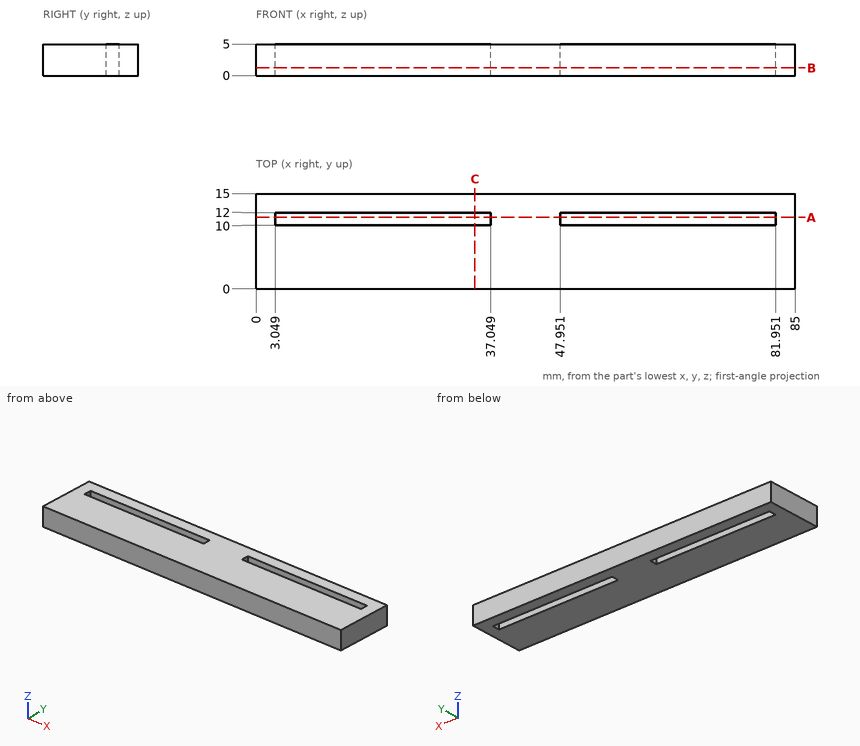
Job drawing, mm, ordinate dimensions from the low corner. One solid piece. Give positions to 0.01 mm unless a question says otherwise; leave off trailing zeros. Write each loop counter-clockwise with the first axis right and the second up, starting at its lowest first coordinate (ties: lowest second). Pieces come first, ordered by that corner, then holes. Notation, with made-up numbers: M 74.25,-35 L 90.25,-35 A22 ccw 90.25,-17 Z; hole C 22.5,65.5 d9. An arc over 180 degrees is marked long. Put each result on its own line as item: value. Start each with the question number.
(1) Band-saw the part on A-A, the plane y = 11.25. Write the cut outline in (x, z).
(2) Band-saw the part on B-B, the plane z = 1.25. Write the cut outline in (x, y).
(3) Band-saw the part on C-C, the plane x = 34.5. Write the cut outline in (y, z).
(4) Probe L1, parallel to X at y = 10.75, z = 0.7; L2, parallel to Y at x = 65, z = 1.65. List the from-to ranges inside material, lowest first.
Response values:
1. outline: M 0,0 L 3.05,0 L 3.05,5 L 0,5 Z; M 37.05,0 L 47.95,0 L 47.95,5 L 37.05,5 Z; M 81.95,0 L 85,0 L 85,5 L 81.95,5 Z
2. outline: M 0,0 L 85,0 L 85,15 L 0,15 Z; hole M 3.05,10 L 37.05,10 L 37.05,12 L 3.05,12 Z; hole M 47.95,10 L 81.95,10 L 81.95,12 L 47.95,12 Z
3. outline: M 0,0 L 10,0 L 10,5 L 0,5 Z; M 12,0 L 15,0 L 15,5 L 12,5 Z
4. L1: x = 0 to 3.05, 37.05 to 47.95, 81.95 to 85
4. L2: y = 0 to 10, 12 to 15
